Can you work these out from the model? Positions are in its coordinate system, mm. Face numbers are marked on the shaded views. A direction names the side the tool comes from. Round coordinates to 2 decimals unless told otherwise and drop trailing zeros. Loops run counter-clockwise (first coordinate to the right, second up) from the corner with the lowest first, then second, coordinate; pieces in that order, holes last. Notation, with made-up numbers: M 4.25,-2.5 L 62.25,-2.5 A15 cw 62.25,3.5 Z; hole C -18.5,51.5 d5. An arc over 180 degrees is marked long. Use a Markdown table: item, result. Add a question column.
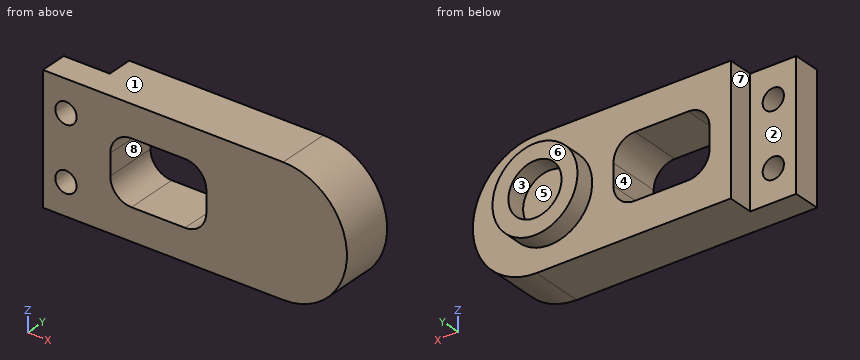
```python
from build123d import *

# Parameters (mm, degrees)
BOSS_EXTRUDE1_DEPTH = 5
SKETCH2_W           = 4.33
SKETCH2_H           = 12
CUT_EXTRUDE1_DEPTH  = 2.42
SKETCH3_R           = 1
CUT_EXTRUDE2_DEPTH  = 3.58
SKETCH5_R           = 4
SKETCH5_R_2         = 2.5
BOSS_EXTRUDE2_DEPTH = 1.83
CUT_EXTRUDE3_DEPTH  = 6


with BuildPart() as part:
    # Sketch1 → Boss-Extrude1 (new body)
    with BuildSketch(Plane(origin=(0, 0, 0), x_dir=(1, 0, 0), z_dir=(0, 1, 0))):
        with BuildLine():
            Line((0, 0), (22.6, 0))
            ThreePointArc((22.6, 0), (28.6, 6), (22.6, 12))
            Line((22.6, 12), (0, 12))
            Line((0, 12), (0, 0))
        make_face()
    extrude(amount=BOSS_EXTRUDE1_DEPTH)

    # Sketch2 → Cut-Extrude1 (cut)
    with BuildSketch(Plane(origin=(0, 5, 0), x_dir=(1, 0, 0), z_dir=(0, 1, 0))):
        with Locations((2.165, 6)):
            Rectangle(SKETCH2_W, SKETCH2_H)
    extrude(amount=-CUT_EXTRUDE1_DEPTH, mode=Mode.SUBTRACT)

    # Sketch3 → Cut-Extrude2 (cut, through all)
    with BuildSketch(Plane(origin=(0, 2.58, 0), x_dir=(1, 0, 0), z_dir=(0, 1, 0))):
        with Locations((2.16, 9)):
            Circle(SKETCH3_R)
        with Locations((2.16, 3)):
            Circle(SKETCH3_R)
    extrude(amount=-CUT_EXTRUDE2_DEPTH, mode=Mode.SUBTRACT)

    # Sketch5 → Boss-Extrude2 (add)
    with BuildSketch(Plane(origin=(0, 5, 0), x_dir=(1, 0, 0), z_dir=(0, 1, 0))):
        with Locations((21.37, 6)):
            Circle(SKETCH5_R)
        with Locations((21.37, 6)):
            Circle(SKETCH5_R_2, mode=Mode.SUBTRACT)
    extrude(amount=BOSS_EXTRUDE2_DEPTH)

    # Sketch6 → Cut-Extrude3 (cut, through all)
    with BuildSketch(Plane(origin=(0, 5, 0), x_dir=(1, 0, 0), z_dir=(0, 1, 0))):
        with BuildLine():
            Line((8.33, 9), (13.37, 9))
            ThreePointArc((13.37, 9), (14.784213562, 8.414213562), (15.37, 7))
            Line((15.37, 7), (15.37, 5))
            ThreePointArc((15.37, 5), (14.784213562, 3.585786438), (13.37, 3))
            Line((13.37, 3), (8.33, 3))
            ThreePointArc((8.33, 3), (6.915786438, 3.585786438), (6.33, 5))
            Line((6.33, 5), (6.33, 7))
            ThreePointArc((6.33, 7), (6.915786438, 8.414213562), (8.33, 9))
        make_face()
    extrude(amount=-CUT_EXTRUDE3_DEPTH, mode=Mode.SUBTRACT)


solid = part.part
```
(1) Suppose I cut it at C-C on x = 2.16. List the corners of the cut face in (y, z) for me.
(2) Suppose I cut it at D-D on y = 5.5. List the corners of the cut face in (x, z) for me.
(3) On a 3-axis mill with a long thin cutter (end or side, diameter ignored), from which of +Z, -Z, +X, -X, +Y, -Y can I reach the whole of each face in a straight line? I mean the marked faces 1, 2, 3 and 4. Say none if no direction works.
(4) I'm going to push flat-ended pins straight in: pin 1 (1.3 mm diameter, centred on x = 2, z = -5, fed in from +Y); pin 2 (1 mm diameter, centred on y = 4.5, z = -2, fed in from +X); pin 3 (3.5 mm diameter, centred on x = 14.5, z = -7.5, fed in from +Y); pin 4 (1 mm diameter, centred on x = 21, z = -9, fed in from -Y). Where does each tip first touch, or does it pass through?
(5) Suppose I cut it at A-A on z = -6. List the corners of the cut face in (x, y) for me.
(6) If I drill on probe 1 along Z at (x, y) = (2.16, 1); probe 2 along X at (y, z) = (6.3, -6); probe 3 along Z at (x, y) = (21.37, 5.65), over which ranges is the centre line in solid material (lowest first)? Write a range as [from, to].
(7) Suppose I cut it at B-B on x = 12.25. List the corners of the cut face in (y, z) for me.
(8) Thinking about a two-plate mould opening in X: for the marked faces 5, 6, 7 and 8, which applies, released by +X, released by -X, zero draft, split by the parting line, or undercut?
Results below:
| question | item | result |
|---|---|---|
| 1 | outline | M 0,-12 L 2.58,-12 L 2.58,-10 L 0,-10 Z; M 0,-8 L 2.58,-8 L 2.58,-4 L 0,-4 Z; M 0,-2 L 2.58,-2 L 2.58,0 L 0,0 Z |
| 2 | outline | C 21.37,-6 d8; hole C 21.37,-6 d5 |
| 3 | face 1 | +Z, +X, -X, +Y, -Y |
| 3 | face 2 | +Z, -Z, -X, +Y |
| 3 | face 3 | +Y |
| 3 | face 4 | +Y, -Y |
| 4 | pin 1 | stops at y = 2.58 |
| 4 | pin 2 | stops at x = 27.47 |
| 4 | pin 3 | stops at y = 5 |
| 4 | pin 4 | stops at y = 0 |
| 5 | outline | M 0,0 L 6.33,0 L 6.33,5 L 4.33,5 L 4.33,2.58 L 0,2.58 Z; M 15.37,0 L 28.6,0 L 28.6,5 L 25.37,5 L 25.37,6.83 L 23.87,6.83 L 23.87,5 L 18.87,5 L 18.87,6.83 L 17.37,6.83 L 17.37,5 L 15.37,5 Z |
| 6 | probe 1 | z = [-12, -10], [-8, -4], [-2, 0] |
| 6 | probe 2 | x = [17.37, 18.87], [23.87, 25.37] |
| 6 | probe 3 | z = [-10, -8.5], [-3.5, -2] |
| 7 | outline | M 0,-12 L 5,-12 L 5,-9 L 0,-9 Z; M 0,-3 L 5,-3 L 5,0 L 0,0 Z |
| 8 | face 5 | undercut |
| 8 | face 6 | zero draft |
| 8 | face 7 | released by -X |
| 8 | face 8 | undercut |
